Verification items for the finished model (mm, model axes). A direction names the side the tool comes from. Coordinates: 2 decimals unless noted, no trailing zeros. Loops run counter-clockwise (first coordinate to the right, second up) from the corner with the lowest first, then second, coordinate; pieces in that order, holes last. Notation, with made-up numbers: (76.5, -36) -> (90.5, -36) arc R14 ccw to (90.5, -14) -> close; hole circle Ø4 at (24, 87). An arc over 180 degrees is marked (long way). Write item = value, one per line.
```python
from build123d import *

# Parameters (mm, degrees)
SKETCH1_W      = 26
SKETCH1_H      = 12
EXTRUDE1_DEPTH = 3
SKETCH2_R      = 2.25
EXTRUDE2_DEPTH = 4
SKETCH3_W      = 7
SKETCH3_H      = 1
EXTRUDE3_DEPTH = 27


with BuildPart() as part:
    # Sketch1 → Extrude1 (new body)
    with BuildSketch(Plane(origin=(0, 0, 0), x_dir=(1, 0, 0), z_dir=(0, 1, 0))):
        Rectangle(SKETCH1_W, SKETCH1_H)
    extrude(amount=-EXTRUDE1_DEPTH)

    # Sketch2 → Extrude2 (cut, through all)
    with BuildSketch(Plane(origin=(0, 0, 0), x_dir=(1, 0, 0), z_dir=(0, 1, 0))):
        with Locations(Location((-6.25, 0, 0), (0, 0, 270))):  # turned: the seam where the file's is
            Circle(SKETCH2_R)
        with Locations(Location((6.25, 0, 0), (0, 0, 270))):  # turned: the seam where the file's is
            Circle(SKETCH2_R)
    extrude(amount=-EXTRUDE2_DEPTH, mode=Mode.SUBTRACT)

    # Sketch3 → Extrude3 (cut, through all)
    with BuildSketch(Plane(origin=(13, 0, 0), x_dir=(0, 0, -1), z_dir=(1, 0, 0))):
        with Locations((0, -2.5)):
            Rectangle(SKETCH3_W, SKETCH3_H)
    extrude(amount=-EXTRUDE3_DEPTH, mode=Mode.SUBTRACT)


solid = part.part
```
1) Material ranges on line 1 (X direction, y = -1.2, z = 0); line 2 (X direction, y = -1.7, z = -0.5); line 3 (Y direction, x = -9.5, z = 0.5), recorded low to high.
Ans:
line_1 = -13 to -8.5, -4 to 4, 8.5 to 13
line_2 = -13 to -8.44, -4.06 to 4.06, 8.44 to 13
line_3 = -2 to 0
2) Release check for a two-part mould opening along X. For faces 1 (the face through (13, -1, 0)), 2 (the face through (0, -1, 6)), 3 (the face through (6.926, -0.986, 2.146)), 4 (the face through (-4, -1, 0)) record: pulls with the +X half, pulls with the -X half, needs draft (parallel to the pull), parting line crosses it, or undercut.
Ans:
face_1 = pulls with the +X half
face_2 = needs draft
face_3 = undercut
face_4 = undercut
3) Tool access check on faces 5 (the face through (0, -2, 0)), 6 (the face through (0, -1, -6)). Record the directions out of +Z, -Z, +X, -X, +Y, -Y that give a thin tool (end or side, any length) a straight path to the whole face; none if there is none.
Ans:
face_5 = +X, -X, -Y
face_6 = -Z, +X, -X, +Y, -Y
4) Sectioned sample at C-C, the plane x = 9.75. Record the cut outline in (y, z).
Ans:
outline = (-3, -6) -> (0, -6) -> (0, 6) -> (-3, 6) -> (-3, 3.5) -> (-2, 3.5) -> (-2, -3.5) -> (-3, -3.5) -> close
5) Sectioned sample at A-A, the plane z = 0. Record the cut outline in (x, y), plus the area to 3 significant figures.
Ans:
outline = (-13, -2) -> (-8.5, -2) -> (-8.5, 0) -> (-13, 0) -> close; (-4, -2) -> (4, -2) -> (4, 0) -> (-4, 0) -> close; (8.5, -2) -> (13, -2) -> (13, 0) -> (8.5, 0) -> close
area = 34.0 mm2
6) Depth check by flat-ended pin: pin 1 Ø2 at (x, z) = (-8.5, -5) entering from +Y; pin 2 Ø2 at (x, z) = (6.5, -0.5) entering from -Y. Enter the tip coordinate at first touch or a pass-through.
Ans:
pin_1 = 0
pin_2 = through
7) Sectioned sample at B-B, the plane x = 6.25. Record the cut outline in (y, z), plus the area to 3 significant figures.
Ans:
outline = (-3, -6) -> (0, -6) -> (0, -2.25) -> (-2, -2.25) -> (-2, -3.5) -> (-3, -3.5) -> close; (-3, 3.5) -> (-2, 3.5) -> (-2, 2.25) -> (0, 2.25) -> (0, 6) -> (-3, 6) -> close
area = 20.0 mm2
8) Sectioned sample at D-D, the plane y = -1.05. Record the cut outline in (x, z), plus the area to 3 significant figures.
Ans:
outline = (-13, -6) -> (13, -6) -> (13, 6) -> (-13, 6) -> close; hole circle Ø4.5 at (-6.25, 0); hole circle Ø4.5 at (6.25, 0)
area = 280 mm2
